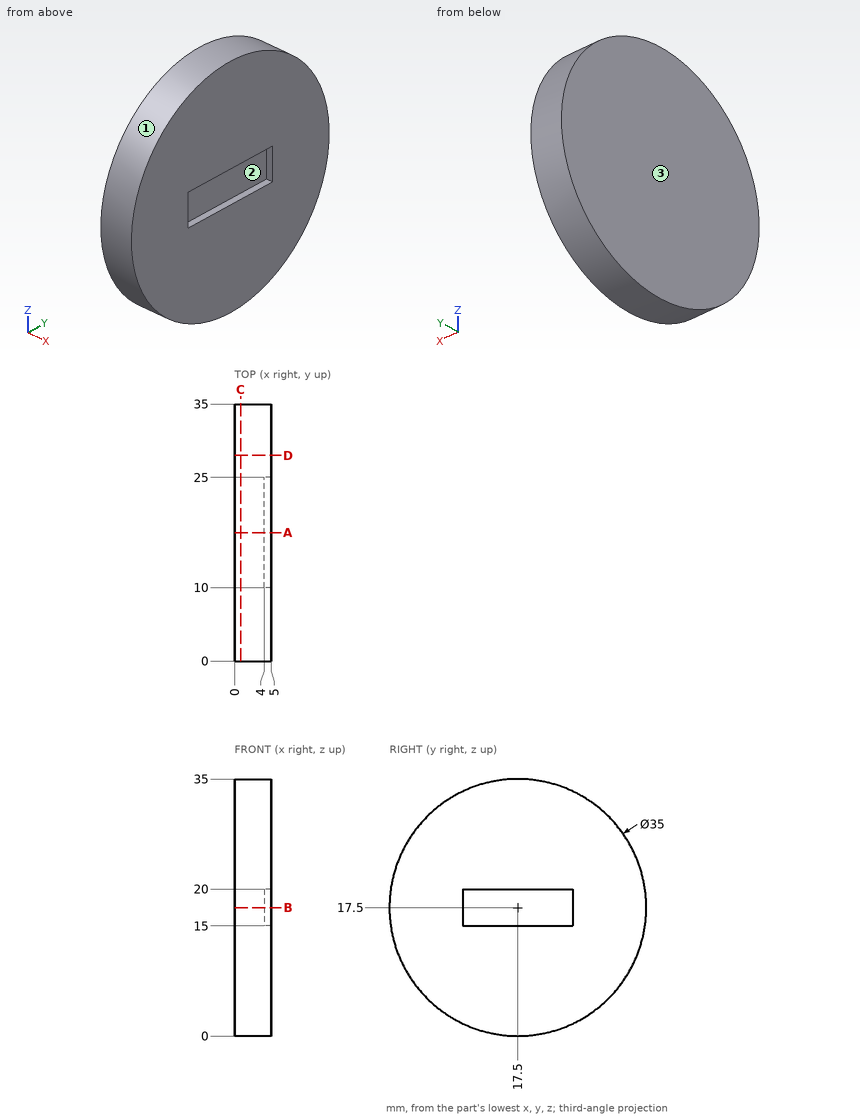
Design review of the part shown in the three views and the two pictorial views. Dimensions are in mm from the part's minimum x, y and z. Coordinates: 2 decimals unless noted, no trailing zeros. Write each loop counter-clockwise with the first axis right and the second up, starting at its lowest first coordinate (ties: lowest second). Pieces come first, ordered by that corner, then holes.
1) We need section D-D on y = 28. State the section outline as (x, z) points.
2) To check wall thickness, follow probe 1 along Z at (x, y) = (3.95, 32); probe 2 along Z at (x, y) = (3.85, 7); probe 3 along Y at (x, z) = (3, 24.5). State the ranges of each line that lie inside material, in increasing order.
3) We need section C-C on x = 0.8. State the section outline as (y, z) points, then the cut area to 3 significant figures.
4) We need section B-B on z = 17.5. State the section outline as (x, y) points, then the cut area to 3 significant figures.
5) We need section A-A on y = 17.5. State the section outline as (x, z) points.
6) Clearance check with flat-ended pins moving along their axes: pin 1 Ø1 at (x, z) = (1, 26) entering from -Y; pin 2 Ø1.1 at (x, z) = (4.5, 16.5) entering from +Y; pin 3 Ø2 at (x, y) = (3.5, 6.5) entering from +Z. State where each tip first meets the part, or that it passes through.
7) The part is to be moulded in two halves that separate along Z. For the marked faces 1, 2 and 3, say which applies: pulls with the +Z half, pulls with the -Z half, needs draft (parallel to the pull), parting line crosses it, or undercut.
Answer list:
1. outline: (0, 3.5) - (5, 3.5) - (5, 31.5) - (0, 31.5) - close
2. probe 1: z = 7.7 to 27.3
2. probe 2: z = 3.5 to 31.5
2. probe 3: y = 1.46 to 33.54
3. outline: circle Ø35 at (17.5, 17.5)
3. area: 962 mm2
4. outline: (0, 0) - (5, 0) - (5, 10) - (4, 10) - (4, 25) - (5, 25) - (5, 35) - (0, 35) - close
4. area: 160 mm2
5. outline: (0, 0) - (5, 0) - (5, 15) - (4, 15) - (4, 20) - (5, 20) - (5, 35) - (0, 35) - close
6. pin 1: stops at y = 1.94
6. pin 2: stops at y = 34.99
6. pin 3: stops at z = 31.86
7. face 1: parting line crosses it
7. face 2: undercut
7. face 3: needs draft
